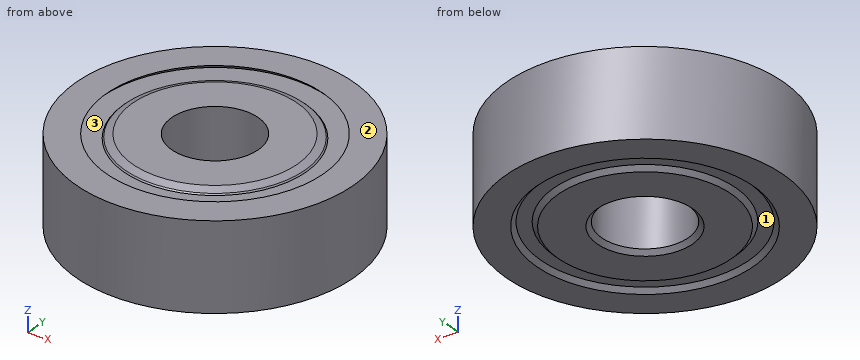
from build123d import *

# Parameters (mm, degrees)
CHAMFER_SIZE = 0.25


with BuildPart() as part:
    # Sketch → Revolution (revolve)
    with BuildSketch(Plane.XZ):
        Polygon((2.5, -2.5), (5, -2.5), (5.25, -2.25), (6, -2.25), (6.25, -2.5), (8, -2.5), (8, 2.5), (6.25, 2.5), (6.5, 2.25), (5.25, 2.25), (5, 2.5), (2.5, 2.5), align=None)
    revolve(axis=Axis((0, 0, 0), (0, 0, 1)))

    # Chamfer
    chamfer_edges = [part.edges().sort_by_distance(p)[0] for p in [
        (-5, 0, 2.5),
        (-2.5, 0, -2.5),
    ]]
    chamfer(chamfer_edges, length=CHAMFER_SIZE)


solid = part.part
Can you work these out from the model? Positions are in its coordinate system, mm. Face numbers are marked on the shaded views. Round coordinates to 2 decimals unless told otherwise and drop trailing zeros. Order: outer loops, then holes, each group sorted by start corner. A loop starts at its lowest first (then second) coordinate and runs counter-clockwise, first axis right, second up. Notation, with made-up numbers: M 66,32 L 94,32 A19 ccw 94,55 Z; hole C 5.5,-18 d8. An arc over 180 degrees is marked long. Use a Markdown table: item, result.
1) If I drill on line 1 along Y through (x, z) = (0, 0.75); line 2 along Y through (x, z) = (0.75, -0.4); line 3 along X through (y, z) = (-2, -1.45), over which ranges is the centre line in solid material (lowest first)?
Geometry says:
| item | result |
|---|---|
| line 1 | y = -8 to -2.5, 2.5 to 8 |
| line 2 | y = -7.96 to -2.38, 2.38 to 7.96 |
| line 3 | x = -7.75 to -1.5, 1.5 to 7.75 |
2) If we mould it in two halves opening along Z, with no side actions, what happens to the marked faces 1, 2 and 3? For each: +Z half, -Z half, draft (parallel to the pull), parting line (faces both ways), or undercut.
Geometry says:
| item | result |
|---|---|
| face 1 | -Z half |
| face 2 | +Z half |
| face 3 | undercut |
3) I'm going to push flat-ended pins straight in: P1, Ø3, axis at x = 0, y = 0, coming from the +Z side; P2, Ø2, axis at x = 4, z = 1, coming from the +Y side; P3, Ø1, axis at y = 1.5, z = -2, coming from the -X side. Where does each tip first touch, or does it pass through?
Geometry says:
| item | result |
|---|---|
| P1 | passes through |
| P2 | stops at y = 7.42 |
| P3 | stops at x = -7.94 |
4) Imagine slicing it at A-A (x = 0). List the corners of the cut face in (y, z) for me, then the cut area to 3 significant figures.
Geometry says:
| item | result |
|---|---|
| outline | M -8,-2.5 L -6.25,-2.5 L -6,-2.25 L -5.25,-2.25 L -5,-2.5 L -2.75,-2.5 L -2.5,-2.25 L -2.5,2.5 L -4.75,2.5 L -5.18,2.32 L -5.25,2.25 L -6.5,2.25 L -6.25,2.5 L -8,2.5 Z; M 2.5,-2.25 L 2.75,-2.5 L 5,-2.5 L 5.25,-2.25 L 6,-2.25 L 6.25,-2.5 L 8,-2.5 L 8,2.5 L 6.25,2.5 L 6.5,2.25 L 5.25,2.25 L 5.18,2.32 L 4.75,2.5 L 2.5,2.5 Z |
| area | 53.8 mm² |
5) Imagine slicing it at C-C (z = -1.6). List the corners of the cut face in (x, y) for me.
Geometry says:
| item | result |
|---|---|
| outline | C 0,0 d16; hole C 0,0 d5 |
